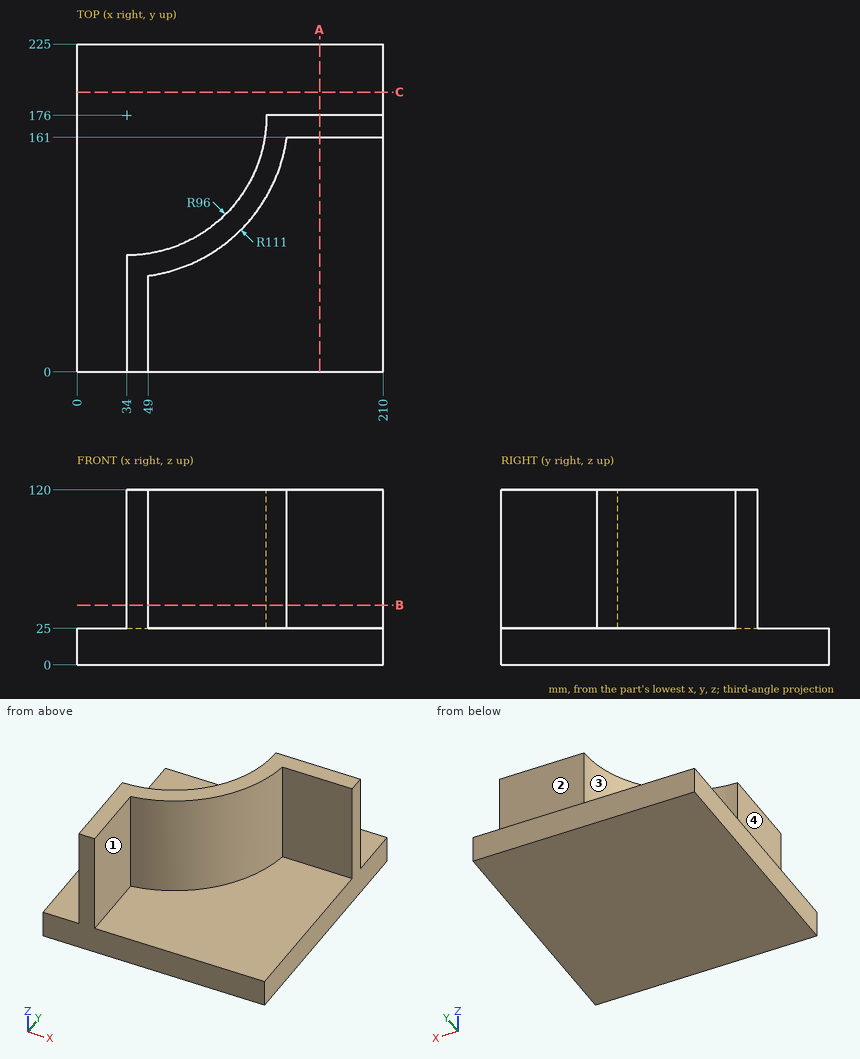
Study the drawing (mm; zero at the part's minimum x, y, z) and answer. A direction names the side the tool comes from. Give positions to 0.01 mm unless a question says otherwise; leave off trailing zeros. Write each loop counter-clockwise with the first axis right and the second up, starting at its lowest first coordinate (ties: lowest second). Pieces come first, ordered by that corner, then holes. Notation, with made-up numbers: (69.25, 85) -> (90.25, 85) arc R10 cw to (90.25, 101) -> close; hole circle Ø11 at (-33, -20). An arc over 180 degrees is marked (long way). Write item = value, one per line. Start each with the question number.
1) Which of the six approach directions +Z, -Z, +X, -X, +Y, -Y give full straight-line access (tool end or side, diameter ignored) to the marked faces 1, 2, 3 and 4?
2) The part is cut by section B-B, the plane z = 41. Determine the outline of the cut face in (x, y).
3) The part is cut by section C-C, the plane y = 192. Determine the outline of the cut face in (x, z), and give its area (3 significant figures).
4) The part is cut by section A-A, the plane x = 166.5. Determine the outline of the cut face in (y, z), and give its area (3 significant figures).
5) Each of these flat-tipped pins is pushed along its axis until it touches: pin 1 (24 mm diameter, centred on y = 35.5, z = 73.5, fed in from -X); pin 2 (1 mm diameter, centred on x = 126, y = 30.5, fed in from +Z); pin 3 (24 mm diameter, centred on x = 175.5, z = 64, fed in from +Y). Where does it stop, or does it pass through?
6) Straight lines are drawn through the part: line 1 along Z through (x, y) = (59, 37); line 2 along Y through (x, z) = (192, 26); line 3 along X through (y, z) = (166, 51.5). For each, find the intervals that lie inside material, in ascending order.
Solutions:
q1.face_1 = +Z, +X, -Y
q1.face_2 = +Z, +X, -X, +Y
q1.face_3 = +Z, -X, +Y
q1.face_4 = +Z, -X, +Y, -Y
q2.outline = (34, 0) -> (49, 0) -> (49, 66.02) arc R111 ccw to (143.98, 161) -> (210, 161) -> (210, 176) -> (130, 176) arc R96 cw to (34, 80) -> close
q3.outline = (0, 0) -> (210, 0) -> (210, 25) -> (0, 25) -> close
q3.area = 5,250 mm²
q4.outline = (0, 0) -> (225, 0) -> (225, 25) -> (176, 25) -> (176, 120) -> (161, 120) -> (161, 25) -> (0, 25) -> close
q4.area = 7,050 mm²
q5.pin_1 = 34
q5.pin_2 = 25
q5.pin_3 = 176
q6.line_1 = 0 to 25
q6.line_2 = 161 to 176
q6.line_3 = 129.48 to 210
